Can you work these out from the model? Positions are in its coordinate system, mm. A direction names the side the tool comes from. Coordinates: 2 decimals unless noted, no trailing zeros. Order: outer loops, then holes, each group sorted by start corner. A loop starts at its lowest first (then second) coordinate and runs counter-clockwise, first axis right, second up. Notation, with made-up numbers: M 52,-14.5 L 69,-14.5 A14 cw 69,1.5 Z; hole C 70,16.5 d4. An arc over 180 degrees is marked long. Answer as CSV lines item,"result". Start each with the question number.
1. On a 3-axis mill with a long thin cutter (end or side, diameter ignored), from which of +Z, -Z, +X, -X, +Y, -Y can I reach the whole of each face in a straight line? I mean faces 1 (the face through (-14, 1, -7)), 2 (the face through (-43, 1, -14)), 3 (the face through (-50, 1, -30)). Say none if no direction works.
2. If we section it at A-A (z = -3.5): List the corners of the cut face in (x, y) for me, plus the area to 3 significant figures.
3. If we section it at B-B (y = 1): List the corners of the cut face in (x, z) for me, plus the area to 3 significant figures.
4. If we section it at C-C (x = -4): List the corners of the cut face in (y, z) for me, plus the area to 3 significant figures.
5. Will these pins go through, and if not, where does the flat tip stop? pin 1 (0.6 mm diameter, centred on y = 1, z = -9.5, fed in from -X); pin 2 (0.6 mm diameter, centred on x = -9.5, y = 0.5, fed in from +Z).
6. I need wall thicknesses on line 1 along X through (y, z) = (1.2, -11); line 2 along Z through (x, y) = (-28, 1); line 3 along Z through (x, y) = (-37, 1.8). Which ranges of each line are inside material? Lowest first, please. Write a range as from..to.
Autodesk Inventor part; units mm, degrees
ref_plane "YZ Plane" through (0, 0, 0) normal (1, 0, 0) x (0, 1, 0)
ref_plane "XZ Plane" through (0, 0, 0) normal (0, 1, 0) x (-1, 0, 0)
ref_plane "XY Plane" through (0, 0, 0) normal (0, 0, 1) x (1, 0, 0)
sketch "Szkic1" plane through (0, 0, 0) normal (0, 1, 0) x (-1, 0, 0)
  line L0 (0, 0) -> (50, 0)
  line L1 (50, 0) -> (50, -50)
  line L2 (50, -50) -> (0, -50)
  line L3 (0, -50) -> (0, 0)
  dimension "d0" = 50
  dimension "d1" = 50
extrude "Wyciągnięcie proste1" add sketch "Szkic1" along normal blind 2
sketch "Szkic2" plane through (0, 2, 0) normal (0, 1, 0) x (1, 0, 0)
  line L0 (0, 50) -> (-50, 50)
  line L1 (-50, 50) -> (-50, 0)
  line L2 (-50, 0) -> (0, 0)
  line L3 (0, 0) -> (0, 50)
  line L4 (0, 0) -> (-14, 0)
  line L5 (-14, 0) -> (-14, 14)
  line L6 (-14, 14) -> (0, 14)
  line L7 (0, 14) -> (0, 0)
  line L8 (-50, 0) -> (-36, 0)
  line L9 (-36, 0) -> (-36, 14)
  line L10 (-36, 14) -> (-50, 14)
  line L11 (-50, 14) -> (-50, 0)
  point P0 (-36, 0)
  point P1 (0, 14)
  point P2 (-14, 0)
  dimension "d4" = 14
  dimension "d5" = 14
  dimension "d8" = 14
  dimension "d11" = 14
extrude "Wyciągnięcie proste2" cut sketch "Szkic2" against normal through all contours L3 L2 L5 L6 | L10 L9 L2 L1
sketch "Szkic4" plane through (-50, 0, -50) normal (-1, 0, 0) x (0, 0, 1)
  line L0 (36, 0) -> (36, 2)
  line L1 (0, 2) -> (36, 2)
  line L2 (0, 0) -> (0, 2)
  line L3 (0, 0) -> (36, 0)
  line L4 (7.6305, -16.85) -> (2.0706, 3.9)
  line L5 (2.0706, 3.9) -> (0, 3.9)
  line L6 (0, 3.9) -> (5.5599, -16.85)
  line L7 (5.5599, -16.85) -> (7.6305, -16.85)
  point P0 (50, 0)
  point P1 (3.1156, 0)
  point P2 (2.5797, 2)
extrude "Wyciągnięcie proste4" cut sketch "Szkic4" against normal through all contours L3 L6 L1 L4 | L3 L2 L1 L6
properties part number "spod" material "Stal, węglowa"
Solved:
1,face 1,"+Z, +X, +Y, -Y"
1,face 2,"+Z, -X, +Y, -Y"
1,face 3,"+Z, -Z, -X, +Y, -Y"
2,outline,"M -36,0 L -14,0 L -14,2 L -36,2 Z"
2,area,"44.0 mm²"
3,outline,"M -50,-47.15 L 0,-47.15 L 0,-14 L -14,-14 L -14,0 L -36,0 L -36,-14 L -50,-14 Z"
3,area,"1,970 mm²"
4,outline,"M 0,-46.88 L 2,-47.42 L 2,-14 L 0,-14 Z"
4,area,"66.3 mm²"
5,pin 1,"x = -36"
5,pin 2,"z = -14"
6,line 1,"-36..-14"
6,line 2,"-47.15..0"
6,line 3,"-47.37..-14"
